from build123d import *

# Parameters (mm, degrees)
SKETCH1_R           = 5.08
BOSS_EXTRUDE1_DEPTH = 3
SKETCH2_R           = 4.445
BOSS_EXTRUDE2_DEPTH = 5
FILLET2_R           = 2
FILLET3_R           = 0.5
SKETCH3_R           = 3.048
BOSS_EXTRUDE3_DEPTH = 6.35
SKETCH4_W           = 1.587384834
SKETCH4_H           = 1.489913834
CUT_EXTRUDE1_DEPTH  = 1.27


with BuildPart() as part:
    # Sketch1 → Boss-Extrude1 (new body)
    with BuildSketch(Plane(origin=(0, 0, 0), x_dir=(1, 0, 0), z_dir=(0, 1, 0))):
        with Locations(Location((0, 0, 0), (0, 0, 270))):
            Circle(SKETCH1_R)
    extrude(amount=BOSS_EXTRUDE1_DEPTH)

    # Sketch2 → Boss-Extrude2 (add)
    with BuildSketch(Plane(origin=(0, 3, 0), x_dir=(1, 0, 0), z_dir=(0, 1, 0))):
        with Locations(Location((0, 0, 0), (0, 0, 270))):
            Circle(SKETCH2_R)
    extrude(amount=BOSS_EXTRUDE2_DEPTH)

    # Fillet2
    # the kernel refuses this fillet: 2 mm, written as the material it takes off along each edge
    with BuildSketch(Plane(origin=(0, 3, 0), x_dir=(0, 0, 1), z_dir=(-1, 0, 0))) as fillet2_piece_1:
        with BuildLine():
            CenterArc((3.08, -1.461771186), FILLET2_R, 0, 46.960687898)
            Line((4.445, 0), (4.4723, 0.029235424))
            ThreePointArc((4.4723, 0.029235424), (4.7625, 0.04), (5.08, 0.04))
            Line((5.08, 0.04), (5.12, 0))
            Line((5.12, 0), (5.12, -1.461771186))
            Line((5.12, -1.461771186), (5.08, -1.461771186))
        make_face()
    revolve(axis=Axis((0, 3, 0), (0, 1, 0)), mode=Mode.SUBTRACT)

    # Fillet3
    fillet3_edges = [part.edges().sort_by_distance(p)[0] for p in [
        (0, 8, -4.445),
    ]]
    fillet(fillet3_edges, radius=FILLET3_R)

    # Sketch3 → Boss-Extrude3 (add)
    with BuildSketch(Plane.XZ):
        with Locations(Location((0, 0, 0), (0, 0, 270))):
            Circle(SKETCH3_R)
    extrude(amount=BOSS_EXTRUDE3_DEPTH)

    # Sketch4 → Cut-Extrude1 (cut)
    with BuildSketch(Plane.XZ.offset(6.35)):
        Rectangle(SKETCH4_W, SKETCH4_H)
    extrude(amount=-CUT_EXTRUDE1_DEPTH, mode=Mode.SUBTRACT)


solid = part.part
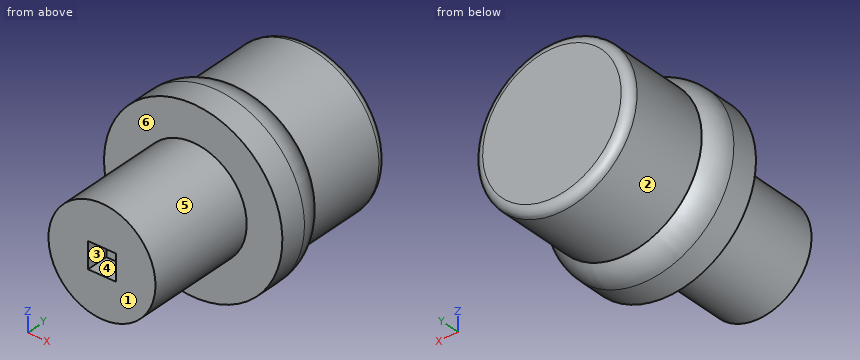
Work out the finished part from the listing and answer in its coordinate system (mm). Face numbers are marked on the shaded views. A direction names the side the tool comes from. Give positions to 0.01 mm unless a question says otherwise; leave off trailing zeros. Order: outer loops, then holes, each group sorted by start corner. A loop starts at its lowest first (then second) coordinate and runs counter-clockwise, first axis right, second up. Notation, with made-up numbers: (-33.5, 79) -> (-23.5, 79) arc R17 cw to (-23.5, 95) -> close; hole circle Ø2 at (-38.75, 44). An arc over 180 degrees is marked (long way). Answer as a JSON object with one key per item and string values. Group by question number.
1. Section D-D on y = 3.5 is taken. Determine the outline of the cut face in (x, z) (3 decimals), plus the area to 3 significant figures.
2. Flat-ended cylindrical pins translate along their axes: pin 1 Ø0.6 at (x, y) = (0, -5.5) entering from -Z; pin 2 Ø1.4 at (y, z) = (-5.5, 0) entering from -X; pin 3 Ø4 at (x, y) = (-3.5, -3) entering from -Z. Find the tip coordinate at first contact, or state that the pin passes through.
3. A tool of negligible diameter and unlimited length cuts with its end or side. For the marked faces 1, 2 and 3, from which of +Z, -Z, +X, -X, +Y, -Y can it reach the whole face along a straight path? Write none if from no direction.
4. Section B-B on z = 0 is taken. Determine the outline of the cut face in (x, y) (3 decimals), plus the area to 3 significant figures.
5. The mould has two halves that part along Z. Classify the marked faces 4, 5 and 6: released by +Z, released by -Z, zero draft, split by the parting line, or undercut.
6. Consider line 1 along Y through (x, z) = (0.75, 3); line 2 along X through (y, z) = (1.25, -3.25); line 3 along Y through (x, z) = (-2.25, -4). Determine where each line is inside the solid, lowest interval first. Write a range as [from, to].
7. Section A-A on x = 0 is taken. Determine the outline of the cut face in (y, z) (3 decimals).
8. Section C-C on y = -4 is taken. Determine the outline of the cut face in (x, z), plus the area to 3 significant figures.
Result sheet:
{
 "1": {"outline": "circle Ø8.89 at (0, 0)", "area": "62.1 mm^2"},
 "2": {"pin 1": "stops at z = -3.05", "pin 2": "stops at x = -3.05", "pin 3": "stops at z = -2.65"},
 "3": {"face 1": "+Z, -Z, +X, -X, -Y", "face 2": "+Y", "face 3": "-Y"},
 "4": {"outline": "(-5.08, 0) -> (-3.048, 0) -> (-3.048, -6.35) -> (-0.794, -6.35) -> (-0.794, -5.08) -> (0.794, -5.08) -> (0.794, -6.35) -> (3.048, -6.35) -> (3.048, 0) -> (5.08, 0) -> (5.08, 1.538) arc R2 ccw to (4.445, 3) -> (4.445, 7.5) arc R0.5 ccw to (3.945, 8) -> (-3.945, 8) arc R0.5 ccw to (-4.445, 7.5) -> (-4.445, 3) arc R2 ccw to (-5.08, 1.538) -> close", "area": "111 mm^2"},
 "5": {"face 4": "undercut", "face 5": "split by the parting line", "face 6": "zero draft"},
 "6": {"line 1": "y = [0, 8]", "line 2": "x = [-3.9, 3.9]", "line 3": "y = [0, 2.85]"},
 "7": {"outline": "(-6.35, -3.048) -> (0, -3.048) -> (0, -5.08) -> (1.538, -5.08) arc R2 ccw to (3, -4.445) -> (7.5, -4.445) arc R0.5 ccw to (8, -3.945) -> (8, 3.945) arc R0.5 ccw to (7.5, 4.445) -> (3, 4.445) arc R2 ccw to (1.538, 5.08) -> (0, 5.08) -> (0, 3.048) -> (-6.35, 3.048) -> (-6.35, 0.745) -> (-5.08, 0.745) -> (-5.08, -0.745) -> (-6.35, -0.745) -> close"},
 "8": {"outline": "circle Ø6.1 at (0, 0)", "area": "29.2 mm^2"}
}
